Can you work these out from the model? Positions are in its coordinate system, mm. Round coordinates to 2 decimals unless told otherwise and drop trailing zeros. Write each loop counter-clockwise with the first axis right and the second up, starting at its lowest first coordinate (ties: lowest second). Pieces come first, ordered by that corner, then holes.
Q1. If we section it at B-B (y = 0): Please give me the cut outline in (x, z), plus the area to 3 significant figures.
Q2. If we section it at A-A (x = 50): Please give me the cut outline in (y, z), plus the area to 3 significant figures.
Q3. If we section it at C-C (x = -15): Please give me the cut outline in (y, z).
Q4. If we section it at D-D (y = 43.5): Please give me the cut outline in (x, z).
Q5. Please list where these lines run through material, in increasing order: line 1 along Y through (x, z) = (-15, 5.5); line 2 along X through (y, z) = (-40, 0.75); line 3 along Y through (x, z) = (57, 4.7).
Autodesk Inventor part; units mm, degrees
ref_plane "YZ Plane" through (0, 0, 0) normal (1, 0, 0) x (0, 1, 0)
ref_plane "XZ Plane" through (0, 0, 0) normal (0, 1, 0) x (-1, 0, 0)
ref_plane "XY Plane" through (0, 0, 0) normal (0, 0, 1) x (1, 0, 0)
sketch "Sketch1" plane through (0, 0, 0) normal (0, 0, 1) x (1, 0, 0)
  line L0 (-70, -55) -> (70, -55)
  line L1 (70, -55) -> (70, 55)
  line L2 (70, 55) -> (-70, 55)
  line L3 (-70, 55) -> (-70, -55)
  line L4 (-70, -55) -> (70, 55) construction
  line L5 (70, -55) -> (-70, 55) construction
  circle A0 centre (50, -35) radius 8.5
  circle A1 centre (50, 35) radius 8.5
  line L6 (0, 0) -> (70, 0) construction
  circle A2 centre (50, 0) radius 8.5
  dimension "d0" = 140
  dimension "d1" = 110
  dimension "d23" = 17
  dimension "d25" = 20
  dimension "d26" = 20
extrude "Plate1" add sketch "Sketch1" along normal blind 6 contours L3 L2 L1 L0 | A0 | A1
sketch "Sketch5" plane through (0, 0, 6) normal (0, 0, 1) x (1, 0, 0)
  line L0 (70, -55) -> (-70, -55)
  line L1 (-70, -55) -> (-70, 55)
  line L2 (-70, 55) -> (70, 55)
  circle A0 centre (-15, 0) radius 55
  circle A1 centre (-15, 0) radius 5
  point P0 (0, 0)
  point P1 (50, -55)
  point P2 (-50, -55)
  point P3 (-70, -35)
  point P4 (-70, 35)
  point P5 (-50, 55)
  point P6 (50, 55)
  dimension "d27" = 10
extrude "Extrusion2" cut sketch "Sketch5" against normal blind 1 contours A1
chamfer "Corner Chamfer2" distance 30 angle 45 2 edges at (70, -55, 3) (70, 55, 3)
fillet "Corner Round2" radius 6 6 edges at (40, -55, 3) (70, -25, 3) (70, 25, 3) (40, 55, 3) (-70, 55, 3) (-70, -55, 3)
equation "\"d26\" = d25"
equation "\"d2\" = Thickness"
equation "\"BendReliefWidth\" = Thickness"
equation "\"BendReliefDepth\" = 0.5 * Thickness"
equation "\"CornerReliefSize\" = 4 * Thickness"
equation "\"MinimumRemnant\" = 2 * Thickness"
equation "\"TransitionRadius\" = BendRadius"
equation "\"JacobiRadiusSize\" = BendRadius"
equation "\"GapSize\" = Thickness"
properties part number "PNS-683 leg floor plate" material "Stainless Steel"
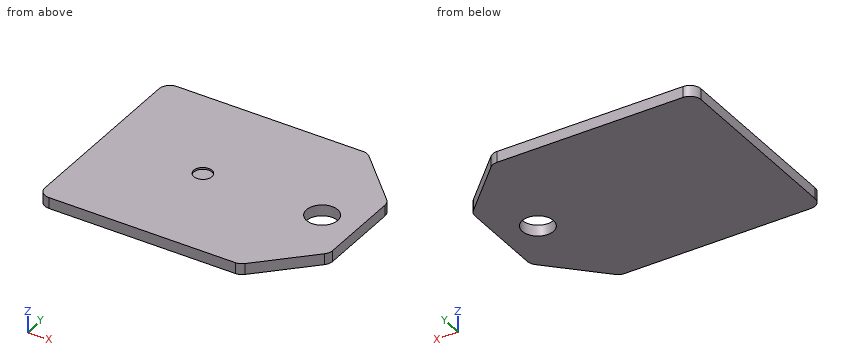
A:
1. outline: (-70, 0) - (41.5, 0) - (41.5, 6) - (-10, 6) - (-10, 5) - (-20, 5) - (-20, 6) - (-70, 6) - close; (58.5, 0) - (70, 0) - (70, 6) - (58.5, 6) - close
1. area: 728 mm2
2. outline: (-45, 0) - (-8.5, 0) - (-8.5, 6) - (-45, 6) - close; (8.5, 0) - (45, 0) - (45, 6) - (8.5, 6) - close
2. area: 438 mm2
3. outline: (-55, 0) - (55, 0) - (55, 6) - (5, 6) - (5, 5) - (-5, 5) - (-5, 6) - (-55, 6) - close
4. outline: (-70, 0) - (51.5, 0) - (51.5, 6) - (-70, 6) - close
5. line 1: y = -55 to -5, 5 to 55
5. line 2: x = -70 to 55
5. line 3: y = -38 to -4.82, 4.82 to 38
